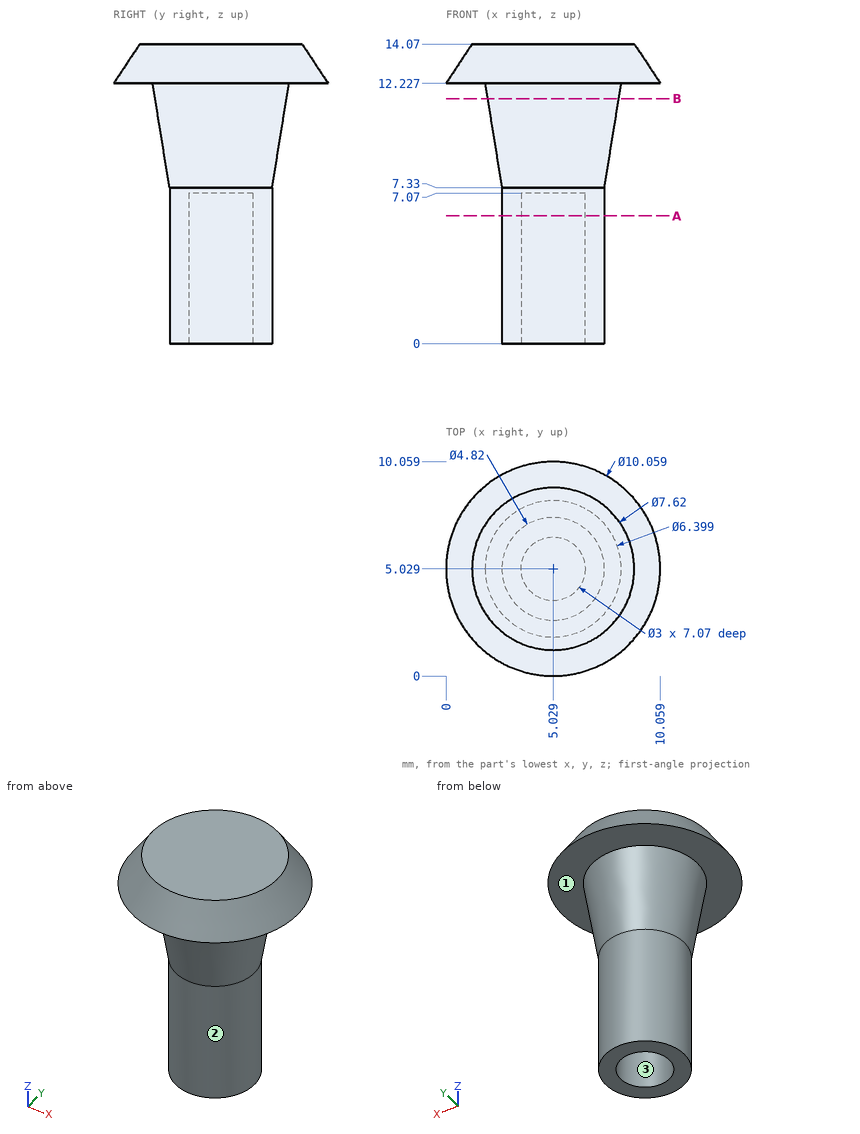
Verification items for this drawing (mm, ordinates from the low corner). Give positions to 0.01 mm unless a question says otherwise; leave off trailing zeros. Write each loop counter-clockwise with the first axis right and the second up, starting at its lowest first coordinate (ties: lowest second). Pieces come first, ordered by that corner, then holes.
1) Section check B-B, the plane z = 11.5. Record the boundary of the cut face in (x, y) (1 decimal).
2) Release check for a two-part mould opening along X. For the marked faces 1, 2 and 3 record: pulls with the +X half, pulls with the -X half, needs draft (parallel to the pull), parting line crosses it, or undercut.
3) Gauge pin test, flat ends, axial feed: pin 1 (1 mm diameter, centred on x = 5, z = 10.5, fed in from -Y); pin 2 (2 mm diameter, centred on y = 4, z = 4, fed in from +X); pin 3 (1 mm diameter, centred on x = 2.5, z = 5, fed in from +Y). Record the tip position at first contact, or that the pin passes through.
4) Material ranges on L1, parallel to Z at x = 1.75, y = 3.75; L2, parallel to X at y = 6, z = 3 (1 decimal); L3, parallel to X at y = 5.5, z = 1.75 (1 decimal), recorded low to high.
5) Section check A-A, the plane z = 6. Record the boundary of the cut face in (x, y).
Computed:
1. outline: circle Ø6.2 at (5, 5)
2. face 1: needs draft
2. face 2: parting line crosses it
2. face 3: undercut
3. pin 1: stops at y = 2.03
3. pin 2: stops at x = 7.44
3. pin 3: stops at y = 6.33
4. L1: z = 12.23 to 14.07
4. L2: x = 2.8 to 3.9, 6.2 to 7.2
4. L3: x = 2.7 to 3.6, 6.5 to 7.4
5. outline: circle Ø4.82 at (5.03, 5.03); hole circle Ø3 at (5.03, 5.03)
